The listing builds one solid part. Answer for the finished solid, in the listing's coordinates (mm). A direction names the side the tool comes from. Give positions to 0.01 mm unless a question says otherwise; leave off trailing zeros. Loops run counter-clockwise (first coordinate to the right, second up) from the corner with the lowest first, then second, coordinate; pieces in that order, holes last.
Item 1: Section C-C, the plane y = 0 is taken. Give the vertices of the cut face in (x, z).
Item 2: Section D-D, the plane y = 4.75 is taken. Give the vertices of the cut face in (x, z).
Item 3: The mould has two halves that part along X. Classify faces 1 (the face through (-4, 6.5, 1)), 2 (the face through (0, -6, 1)), 3 (the face through (1.5, 8, 1)): pulls with the +X half, pulls with the -X half, needs draft (parallel to the pull), parting line crosses it, or undercut.
Item 4: A tool of negligible diameter and unlimited length cuts with its end or side. For faces 4 (the face through (4, 6.5, 1)), 5 (the face through (0, 6, 1)), 6 (the face through (0, 6.4, 0)), 7 (the face through (-1.5, 8, 1)), 8 (the face through (6.5, 0, 1)), from which of +Z, -Z, +X, -X, +Y, -Y can it reach the whole face along a straight path? Write none if from no direction.
Item 5: Section A-A, the plane z = 0.8 is taken. Give the vertices of the cut face in (x, y), and give its area (3 significant figures).
Item 6: Section B-B, the plane x = -4 is taken. Give the vertices of the cut face in (y, z), and give its area (3 significant figures).
Item 7: This flat-tipped pin is pushed along its axis until it touches: pin 1 Ø0.6 at (y, z) = (8.5, 1) entering from -X. Where does it stop, or does it pass through?
Item 8: Consider line 1 along X through (y, z) = (-5.25, 0.45); line 2 along X through (y, z) = (7.25, 0.4). Determine where each line is inside the solid, lowest interval first.
from build123d import *

# Parameters (mm, degrees)
SKETCH_1_W          = 13
SKETCH_1_H          = 13
SKETCH_1_W_2        = 12
SKETCH_1_H_2        = 12
EXTRUDE_1_DEPTH     = 1.2
SKETCH_2_W          = 13
SKETCH_2_H          = 13
SKETCH_2_R          = 4.5
EXTRUDE_2_DEPTH     = 0.1
SKETCH_3_W          = 3
SKETCH_3_H          = 1.3
EXTRUDE_3_DEPTH     = 4
CUT_EXTRUDE_1_DEPTH = 4
SKETCH_5_R          = 1
CUT_EXTRUDE_2_DEPTH = 4


with BuildPart() as part:
    # 草图1 → 凸台-拉伸1 (new body)
    with BuildSketch(Plane.XY):
        Rectangle(SKETCH_1_W, SKETCH_1_H)
        Rectangle(SKETCH_1_W_2, SKETCH_1_H_2, mode=Mode.SUBTRACT)
    extrude(amount=EXTRUDE_1_DEPTH)

    # 草图2 → 凸台-拉伸2 (add)
    with BuildSketch(Plane.XY.offset(1.2)):
        Rectangle(SKETCH_2_W, SKETCH_2_H)
        Circle(SKETCH_2_R, mode=Mode.SUBTRACT)
    extrude(amount=EXTRUDE_2_DEPTH)

    # 草图3 → 凸台-拉伸3 (add)
    with BuildSketch(Plane(origin=(0, 6.5, 0), x_dir=(1, 0, 0), z_dir=(0, 1, 0))):
        with Locations((0, -0.65)):
            Rectangle(SKETCH_3_W, SKETCH_3_H)
    extrude(amount=EXTRUDE_3_DEPTH)

    # 草图4 → 切除-拉伸1 (cut)
    with BuildSketch(Plane.XY.offset(1.3)):
        with BuildLine():
            Line((-1.5, 10.5), (-1.5, 9))
            ThreePointArc((-1.5, 9), (-1.060660172, 10.060660172), (0, 10.5))
            Line((0, 10.5), (-1.5, 10.5))
        make_face()
        with BuildLine():
            ThreePointArc((0, 10.5), (1.060660172, 10.060660172), (1.5, 9))
            Line((1.5, 9), (1.5, 10.5))
            Line((1.5, 10.5), (0, 10.5))
        make_face()
    extrude(amount=-CUT_EXTRUDE_1_DEPTH, mode=Mode.SUBTRACT)

    # 草图5 → 切除-拉伸2 (cut)
    with BuildSketch(Plane.XY.offset(1.3)):
        with Locations((0, 9)):
            Circle(SKETCH_5_R)
    extrude(amount=-CUT_EXTRUDE_2_DEPTH, mode=Mode.SUBTRACT)


solid = part.part
Worked answers:
1. outline: (-6.5, 0) - (-6, 0) - (-6, 1.2) - (-4.5, 1.2) - (-4.5, 1.3) - (-6.5, 1.3) - close; (4.5, 1.2) - (6, 1.2) - (6, 0) - (6.5, 0) - (6.5, 1.3) - (4.5, 1.3) - close
2. outline: (-6.5, 0) - (-6, 0) - (-6, 1.2) - (6, 1.2) - (6, 0) - (6.5, 0) - (6.5, 1.3) - (-6.5, 1.3) - close
3. face 1: needs draft
3. face 2: undercut
3. face 3: pulls with the +X half
4. face 4: +Z, -Z, +X, +Y
4. face 5: -Z
4. face 6: -Z, +X, -X, +Y, -Y
4. face 7: +Z, -Z, -X, +Y
4. face 8: +Z, -Z, +X, +Y, -Y
5. outline: (-6.5, -6.5) - (6.5, -6.5) - (6.5, 6.5) - (1.5, 6.5) - (1.5, 9) arc R1.5 ccw to (-1.5, 9) - (-1.5, 6.5) - (-6.5, 6.5) - close; hole (-6, -6) - (6, -6) - (6, 6) - (-6, 6) - close; hole circle Ø2 at (0, 9)
5. area: 32.9 mm2
6. outline: (-6.5, 0) - (-6, 0) - (-6, 1.2) - (-2.06, 1.2) - (-2.06, 1.3) - (-6.5, 1.3) - close; (2.06, 1.2) - (6, 1.2) - (6, 0) - (6.5, 0) - (6.5, 1.3) - (2.06, 1.3) - close
6. area: 2.09 mm2
7. pin 1: stops at x = -1.5
8. line 1: x = -6.5 to -6, 6 to 6.5
8. line 2: x = -1.5 to 1.5
